Verification items for the finished model (mm, model axes). Face numbers are marked on the shaded views. A direction names the side the tool comes from. Coordinates: 2 decimals unless noted, no trailing zeros. Write each loop counter-clockwise with the first axis right and the second up, starting at its lowest first coordinate (ties: lowest second). Pieces come first, ordered by that corner, then holes. Notation, with made-up numbers: (-3, -1) - (21, -1) arc R27 ccw to (21, 26) - close; hole circle Ø8 at (78, 50.25). An arc over 180 degrees is marked (long way). Use CSV: the item, a comma, the result in double quotes. Start each with the question number.
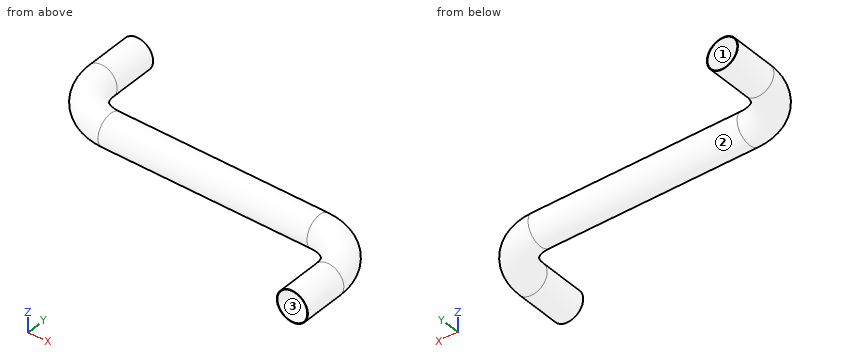
```python
from build123d import *

# Parameters (mm, degrees)
SKETCH1_R   = 26
SKETCH1_R_2 = 25


with BuildPart() as part:
    # Sweep-Thin1: sweep along a path in Sketch2
    with BuildLine(Plane.XY) as sweep_thin1_path:
        Line((0, 0), (0, -75))
        ThreePointArc((0, -75), (21.966991411, -128.033008589), (75, -150))
        Line((75, -150), (425, -150))
        ThreePointArc((425, -150), (478.033008589, -171.966991411), (500, -225))
        Line((500, -225), (500, -300))
    # Sketch1 → Sweep-Thin1 (sweep)
    with BuildSketch(Plane(origin=(0, 0, 0), x_dir=(1, 0, 0), z_dir=(0, 1, 0))):
        Circle(SKETCH1_R)
        Circle(SKETCH1_R_2, mode=Mode.SUBTRACT)
    sweep(path=sweep_thin1_path.line)


solid = part.part
```
Q1. Cross-section at B-B (x = 395). Record the cut outline in (y, z).
Q2. Tool access check on the marked faces 1, 2 and 3. Record the directions out of +Z, -Z, +X, -X, +Y, -Y that give a thin tool (end or side, any length) a straight path to the whole face; none if there is none.
Q3. Cross-section at A-A (z = -9). Record the cut outline in (x, y), plus the area to 3 significant figures.
Q4. Cross-section at C-C (z = 14). Record the cut outline in (x, y).
Q5. Gauge pin test, flat ends, axial feed: pin 1 (2 mm diameter, centred on x = 453.5, y = -173.5, fed in from +Z); pin 2 (8 mm diameter, centred on x = 210, z = 19.5, fed in from +Y); pin 3 (3 mm diameter, centred on x = 373.5, z = -8.5, fed in from +Y). Record the tip position at first contact, or that the pin passes through.
Q6. Scan lines: line 1 along X through (y, z) = (-240, 0); line 2 along X through (y, z) = (-59, -2); line 3 along Y through (x, z) = (365.5, 1). Record each from-to range of solid material in increasing order. Write a range as from..to.
Reply:
1,outline,"circle Ø52 at (-150, 0); hole circle Ø50 at (-150, 0)"
2,face 1,"+Y"
2,face 2,"none"
2,face 3,"-Y"
3,outline,"(-24.39, -75) arc R99.39 ccw to (75, -174.39) - (425, -174.39) arc R50.61 cw to (475.61, -225) - (475.61, -300) - (476.68, -300) - (476.68, -225) arc R51.68 ccw to (425, -173.32) - (75, -173.32) arc R98.32 cw to (-23.32, -75) - (-23.32, 0) - (-24.39, 0) - close; (23.32, -75) arc R51.68 ccw to (75, -126.68) - (425, -126.68) arc R98.32 cw to (523.32, -225) - (523.32, -300) - (524.39, -300) - (524.39, -225) arc R99.39 ccw to (425, -125.61) - (75, -125.61) arc R50.61 cw to (24.39, -75) - (24.39, 0) - (23.32, 0) - close"
3,area,"1,570 mm^2"
4,outline,"(-21.91, -75) arc R96.91 ccw to (75, -171.91) - (425, -171.91) arc R53.09 cw to (478.09, -225) - (478.09, -300) - (479.29, -300) - (479.29, -225) arc R54.29 ccw to (425, -170.71) - (75, -170.71) arc R95.71 cw to (-20.71, -75) - (-20.71, 0) - (-21.91, 0) - close; (20.71, -75) arc R54.29 ccw to (75, -129.29) - (425, -129.29) arc R95.71 cw to (520.71, -225) - (520.71, -300) - (521.91, -300) - (521.91, -225) arc R96.91 ccw to (425, -128.09) - (75, -128.09) arc R53.09 cw to (21.91, -75) - (21.91, 0) - (20.71, 0) - close"
5,pin 1,"z = 21.14"
5,pin 2,"y = -129.13"
5,pin 3,"y = -124.96"
6,line 1,"474..475, 525..526"
6,line 2,"-25.92..-24.92, 24.92..25.92"
6,line 3,"-175.98..-174.98, -125.02..-124.02"
